Geometry: final body of the model. Coordinates: model frame, mm. Coordinates: 2 decimals unless noted, no trailing zeros. Order: outer loops, then holes, each group sorted by start corner. A loop starts at its lowest first (then second) coordinate and runs counter-clockwise, first axis right, second up. Notation, with made-up numbers: (44.5, 41) - (74.5, 41) arc R9 cw to (74.5, 46) - close; hole circle Ø3 at (-4.75, -3.75). An arc over 180 degrees is marked (long way). Use a Markdown table: item, result. Add a question column.
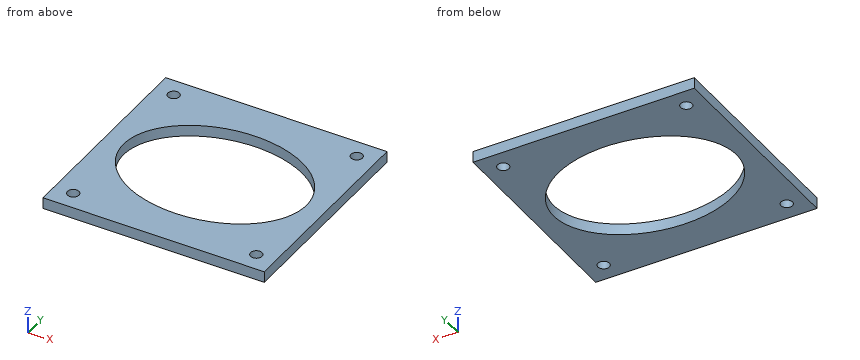
```python
from build123d import *

# Parameters (mm, degrees)
SKETCH1_W           = 115.9
SKETCH1_H           = 110
SKETCH1_R           = 3
SKETCH1_RX          = 47.95
SKETCH1_RY          = 35.45
BOSS_EXTRUDE1_DEPTH = 5.85


with BuildPart() as part:
    # Sketch1 → Boss-Extrude1 (new body)
    with BuildSketch(Plane.XY):
        Rectangle(SKETCH1_W, SKETCH1_H)
        with Locations((-47.95, 45)):
            Circle(SKETCH1_R, mode=Mode.SUBTRACT)
        with Locations((-47.95, -45)):
            Circle(SKETCH1_R, mode=Mode.SUBTRACT)
        with Locations((47.95, -45)):
            Circle(SKETCH1_R, mode=Mode.SUBTRACT)
        with Locations((47.95, 45)):
            Circle(SKETCH1_R, mode=Mode.SUBTRACT)
        with Locations((0, 0)):
            Ellipse(SKETCH1_RX, SKETCH1_RY, mode=Mode.SUBTRACT)
    extrude(amount=BOSS_EXTRUDE1_DEPTH)


solid = part.part
```
1) Section C-C (z = 2). Give the number of separate pieces and of enclosed holes in the cut face, then the cut area to 3 significant figures.
2) Section B-B (x = -49.5). Return loops of the section in (y, z).
3) Ray query, line 1 along Y through (x, z) = (-48, 1.85); line 2 along Y through (x, z) = (-50.5, 5.5); line 3 along X through (y, z) = (-1, 2). Return the intervals inside material, ascending.
4) Section A-A (y = 45). Return loops of the section in (x, z).
5) Pin query (flat end, axial travel): pin 1 (9.5 mm diameter, centred on x = -47.95, y = 45, fed in from +Z). Return the tip coordinate at first contact, or that it passes through.
Values follow:
| question | item | result |
|---|---|---|
| 1 | separate pieces | 1 |
| 1 | enclosed holes | 5 |
| 1 | area | 7,300 mm² |
| 2 | outline | (-55, 0) - (-47.57, 0) - (-47.57, 5.85) - (-55, 5.85) - close; (-42.43, 0) - (42.43, 0) - (42.43, 5.85) - (-42.43, 5.85) - close; (47.57, 0) - (55, 0) - (55, 5.85) - (47.57, 5.85) - close |
| 3 | line 1 | y = -55 to -48, -42 to 42, 48 to 55 |
| 3 | line 2 | y = -55 to -46.58, -43.42 to 43.42, 46.58 to 55 |
| 3 | line 3 | x = -57.95 to -47.93, 47.93 to 57.95 |
| 4 | outline | (-57.95, 0) - (-50.95, 0) - (-50.95, 5.85) - (-57.95, 5.85) - close; (-44.95, 0) - (44.95, 0) - (44.95, 5.85) - (-44.95, 5.85) - close; (50.95, 0) - (57.95, 0) - (57.95, 5.85) - (50.95, 5.85) - close |
| 5 | pin 1 | stops at z = 5.85 |
